Read the model definition and answer for the solid it produces. Units are mm, in the model's axes. Face numbers are marked on the shaded views. A direction names the side the tool comes from. Give positions to 0.01 mm unless a question says otherwise; leave off trailing zeros. Order: outer loops, then holes, each group sorted by start corner. A loop starts at its lowest first (then second) coordinate and runs counter-clockwise, first axis right, second up.
```python
from build123d import *

# Parameters (mm, degrees)
SKETCH1_W           = 60
SKETCH1_H           = 60
BOSS_EXTRUDE1_DEPTH = 10
SKETCH2_R           = 25
BOSS_EXTRUDE2_DEPTH = 5
SKETCH3_R           = 15
BOSS_EXTRUDE3_DEPTH = 35
SKETCH4_R           = 2.5
CUT_EXTRUDE1_DEPTH  = 5
FILLET1_R           = 3
FILLET2_R           = 3
FILLET3_R           = 1


with BuildPart() as part:
    # Sketch1 → Boss-Extrude1 (new body)
    with BuildSketch(Plane(origin=(0, 0, 0), x_dir=(0, 0, -1), z_dir=(1, 0, 0))):
        Rectangle(SKETCH1_W, SKETCH1_H)
    extrude(amount=BOSS_EXTRUDE1_DEPTH)

    # Sketch2 → Boss-Extrude2 (add)
    with BuildSketch(Plane(origin=(10, 0, 0), x_dir=(0, 0, -1), z_dir=(1, 0, 0))):
        Circle(SKETCH2_R)
    extrude(amount=BOSS_EXTRUDE2_DEPTH)

    # Sketch3 → Boss-Extrude3 (add)
    with BuildSketch(Plane(origin=(15, 0, 0), x_dir=(0, 0, -1), z_dir=(1, 0, 0))):
        Circle(SKETCH3_R)
    extrude(amount=BOSS_EXTRUDE3_DEPTH)

    # Sketch4 → Cut-Extrude1 (cut)
    with BuildSketch(Plane(origin=(50, 0, 0), x_dir=(0, 0, -1), z_dir=(1, 0, 0))):
        Circle(SKETCH4_R)
    extrude(amount=-CUT_EXTRUDE1_DEPTH, mode=Mode.SUBTRACT)

    # Fillet1
    fillet1_edges = [part.edges().sort_by_distance(p)[0] for p in [
        (10, 0, 30),
        (10, -30, 0),
        (10, 0, -30),
        (5, -30, -30),
        (5, -30, 30),
        (5, 30, 30),
        (5, 30, -30),
        (10, 30, 0),
    ]]
    fillet(fillet1_edges, radius=FILLET1_R)

    # Fillet2
    fillet2_edges = [part.edges().sort_by_distance(p)[0] for p in [
        (15, 0, 25),
    ]]
    fillet(fillet2_edges, radius=FILLET2_R)

    # Fillet3
    fillet3_edges = [part.edges().sort_by_distance(p)[0] for p in [
        (10, 0, 25),
        (15, 0, 15),
        (50, 0, 15),
    ]]
    fillet(fillet3_edges, radius=FILLET3_R)


solid = part.part
```
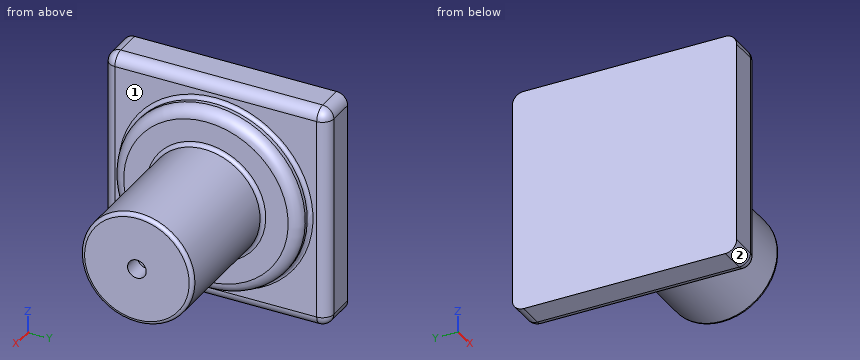
1) A tool of negligible diameter and unlimited length cuts with its end or side. For the marked faces 1 and 2, from which of +Z, -Z, +X, -X, +Y, -Y can it reach the whole face along a straight path? Write none if from no direction.
Final values:
face 1: +X
face 2: -Z, +X, -X, -Y
2) The part is cut by section C-C on x = 36.5. Determine the outline of the cut face in (y, z), and give its area (3 significant figures).
Final values:
outline: circle Ø30 at (0, 0)
area: 707 mm2
3) Consider L1, parallel to Y at x = 47.7, z = 0; L2, parallel to X at y = -2, z = 0; L3, parallel to X at y = 16, z = 12.5. Determine where each line is inside the solid, lowest interval first.
Final values:
L1: y = -15 to -2.5, 2.5 to 15
L2: x = 0 to 45
L3: x = 0 to 15
4) The part is cut by section A-A on y = 0. Determine the outline of the cut face in (x, z).
Final values:
outline: (0, -30) - (7, -30) arc R3 ccw to (10, -27) - (10, -26) arc R1 cw to (11, -25) - (12, -25) arc R3 ccw to (15, -22) - (15, -16) arc R1 cw to (16, -15) - (49, -15) arc R1 ccw to (50, -14) - (50, -2.5) - (45, -2.5) - (45, 2.5) - (50, 2.5) - (50, 14) arc R1 ccw to (49, 15) - (16, 15) arc R1 cw to (15, 16) - (15, 22) arc R3 ccw to (12, 25) - (11, 25) arc R1 cw to (10, 26) - (10, 27) arc R3 ccw to (7, 30) - (0, 30) - close
5) Given pin 1 (1 mm diameter, centred on y = 16.5, z = 4.5, fed in from -X); pin 2 (6 mm diameter, centred on y = -16.5, z = -6.5, fed in from +X); pin 3 (12 mm diameter, centred on x = 18, z = 6, fed in from +Y); pin 4 (12 mm diameter, centred on x = 14.5, y = -14, fed in from -Z), each flat-ended and moving along its own axis, determine where each tip first touches the part or whether it passes through.
Final values:
pin 1: stops at x = 0
pin 2: stops at x = 49.68
pin 3: stops at y = 24.71
pin 4: stops at z = -29.6
